Part model, mm, in its own coordinate system. Face numbers are marked on the shaded views. Coordinates: 2 decimals unless noted, no trailing zeros. Loops run counter-clockwise (first coordinate to the right, second up) from the corner with the lowest first, then second, coordinate; pieces in that order, holes last. Notation, with made-up numbers: M -4,19 L 40,19 A23 cw 40,53 Z; hole C -28,2 d5. An arc over 180 degrees is marked long. Answer as a JSON object with one key per item and string values. Group by question number.
1. Drop a flat-ended pin along its axis: pin 1 Ø3.5 at (x, y) = (0, 0) entering from -Z. Give the stop position or say it passes through.
2. Drill centre lines: L1, parallel to Y at x = 0, z = -0.05; L2, parallel to X at y = -1.25, z = -0.05; L3, parallel to X at y = 2, z = -0.2. Where is each one in solid material? Low to high.
3. Saw through at A-A on y = 0. Write the cut outline in (x, z).
4. Mould opens along X. For the marked faces 1 and 2 say: released by +X, released by -X, zero draft, split by the parting line, or undercut.
5. Saw through at C-C on z = -0.2. Write the cut outline in (x, y), then the cut area to 3 significant figures.
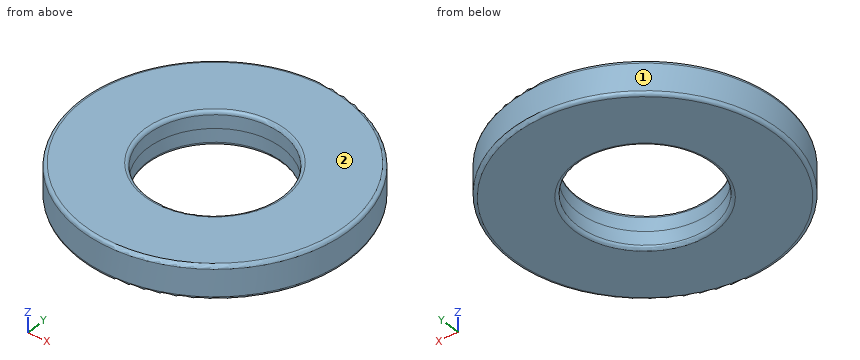
from build123d import *

# Parameters (mm, degrees)
SKETCH3_R                = 6
SKETCH3_R_2              = 3
BOSS_EXTRUDE1_DEPTH      = 0.75
BOSS_EXTRUDE1_DEPTH_BACK = 0.75
FILLET1_R                = 0.15


with BuildPart() as part:
    # Sketch3 → Boss-Extrude1 (new body, two sides)
    with BuildSketch(Plane.XY) as boss_extrude1_sk:
        Circle(SKETCH3_R)
        Circle(SKETCH3_R_2, mode=Mode.SUBTRACT)
    extrude(amount=BOSS_EXTRUDE1_DEPTH)
    extrude(boss_extrude1_sk.sketch, amount=-BOSS_EXTRUDE1_DEPTH_BACK)

    # Fillet1
    fillet1_edges = [part.edges().sort_by_distance(p)[0] for p in [
        (-6, 0, 0.75),
        (-3, 0, 0.75),
        (-6, 0, -0.75),
        (-3, 0, -0.75),
    ]]
    fillet(fillet1_edges, radius=FILLET1_R)


solid = part.part
Outcome:
{
 "1": {"pin 1": "passes through"},
 "2": {"L1": "y = -6 to -3, 3 to 6", "L2": "x = -5.87 to -2.73, 2.73 to 5.87", "L3": "x = -5.66 to -2.24, 2.24 to 5.66"},
 "3": {"outline": "M -6,-0.6 A0.15 ccw -5.85,-0.75 L -3.15,-0.75 A0.15 ccw -3,-0.6 L -3,0.6 A0.15 ccw -3.15,0.75 L -5.85,0.75 A0.15 ccw -6,0.6 Z; M 3,-0.6 A0.15 ccw 3.15,-0.75 L 5.85,-0.75 A0.15 ccw 6,-0.6 L 6,0.6 A0.15 ccw 5.85,0.75 L 3.15,0.75 A0.15 ccw 3,0.6 Z"},
 "4": {"face 1": "split by the parting line", "face 2": "zero draft"},
 "5": {"outline": "C 0,0 d12; hole C 0,0 d6", "area": "84.8 mm²"}
}
